Design review of the part built by this model. Coordinates are the model's own, in mm. Round coordinates to 2 decimals unless told otherwise and drop trailing zeros. Loops run counter-clockwise (first coordinate to the right, second up) from the corner with the lowest first, then second, coordinate; pieces in that order, holes last. Notation, with made-up numbers: (42.5, 6) - (66.5, 6) arc R15 cw to (66.5, 21) - close; hole circle Ø7 at (-0.75, -34.75). An arc over 180 degrees is marked (long way). Use one line per item in the form item = value. Start each with the question number.
(1) We need section B-B, the plane x = 52.5. Write out the cut boundary in (y, z), then the cut area to 3 significant figures.
(2) We need section D-D, the plane y = 1.5. Write out the cut boundary in (x, z).
(3) We need section A-A, the plane z = 45. Write out the cut boundary in (x, y), then the cut area to 3 significant figures.
(4) We need section C-C, the plane x = 0. Write out the cut boundary in (y, z).
(5) For pin 1 (5 mm diameter, centred on x = 52.5, z = 30.31, fed in from +Y); pin 2 (1.5 mm diameter, centred on x = -12.5, y = 2, fed in from -Z); pin 3 (1.5 mm diameter, centred on x = 37.5, y = 0.5, fed in from -Z), all flat-tipped, find the tip position at first contact; note any pin that passes through.
(6) Wall thickness on probe 1 along X at (y, z) = (1.75, -4); probe 2 along Z at (x, y) = (32, 2.35); probe 3 along Z at (x, y) = (-6, 2): over which ranges is each line inside the solid? List them lowest first. Write a range as [from, to].
from build123d import *

# Parameters (mm, degrees)
SKETCH1_R           = 3.05
SKETCH1_R_2         = 4
BOSS_EXTRUDE1_DEPTH = 3


with BuildPart() as part:
    # Sketch1 → Boss-Extrude1 (new body)
    with BuildSketch(Plane(origin=(0, 0, 0), x_dir=(1, 0, 0), z_dir=(0, 1, 0))):
        with BuildLine():
            Line((6.495190528, 64.371778265), (58.995190528, -26.560889132))
            ThreePointArc((58.995190528, -26.560889132), (58.995190528, -34.060889132), (52.5, -37.810889132))
            Line((52.5, -37.810889132), (-52.5, -37.810889132))
            ThreePointArc((-52.5, -37.810889132), (-58.995190528, -34.060889132), (-58.995190528, -26.560889132))
            Line((-58.995190528, -26.560889132), (-6.495190528, 64.371778265))
            ThreePointArc((-6.495190528, 64.371778265), (0, 68.121778265), (6.495190528, 64.371778265))
        make_face()
        with Locations((-52.5, -30.310889132)):
            Circle(SKETCH1_R, mode=Mode.SUBTRACT)
        with Locations((52.5, -30.310889132)):
            Circle(SKETCH1_R, mode=Mode.SUBTRACT)
        with Locations((0, 60.621778265)):
            Circle(SKETCH1_R, mode=Mode.SUBTRACT)
        with BuildLine():
            ThreePointArc((-52.5, -37.810889132), (-53.69003782, -37.715874614), (-54.849923408, -37.433238462))
            Line((-54.849923408, -37.433238462), (-3.133231211, -54.496465773))
            ThreePointArc((-3.133231211, -54.496465773), (0, -55), (3.133231211, -54.496465773))
            Line((3.133231211, -54.496465773), (54.849923408, -37.433238462))
            ThreePointArc((54.849923408, -37.433238462), (53.69003782, -37.715874614), (52.5, -37.810889132))
            Line((52.5, -37.810889132), (-52.5, -37.810889132))
        make_face()
        with Locations((0, -45)):
            Circle(SKETCH1_R_2, mode=Mode.SUBTRACT)
    extrude(amount=BOSS_EXTRUDE1_DEPTH)


solid = part.part
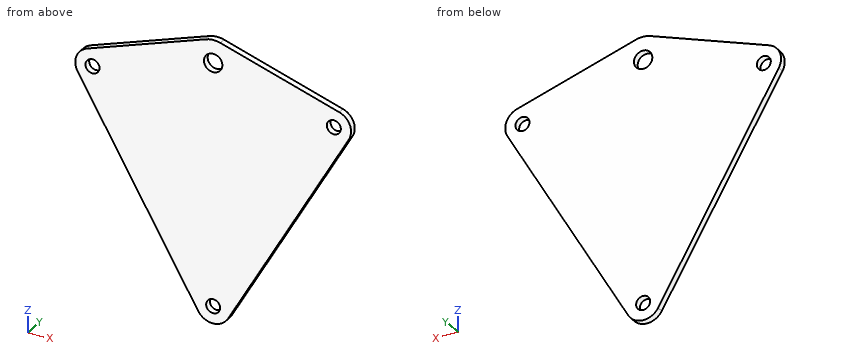
Data:
q1.outline = (0, 15.31) - (3, 15.31) - (3, 27.26) - (0, 27.26) - close; (0, 33.36) - (3, 33.36) - (3, 38.21) - (0, 38.21) - close
q1.area = 50.4 mm^2
q2.outline = (-59, 26.56) - (-6.5, -64.37) arc R7.5 ccw to (6.5, -64.37) - (59, 26.56) arc R7.5 ccw to (54.85, 37.43) - (3.13, 54.5) arc R10 ccw to (-3.13, 54.5) - (-54.85, 37.43) arc R7.5 ccw to start; hole circle Ø6.1 at (-52.5, 30.31); hole circle Ø8 at (0, 45); hole circle Ø6.1 at (0, -60.62); hole circle Ø6.1 at (52.5, 30.31)
q3.outline = (-31.92, 0) - (-4, 0) - (-4, 3) - (-31.92, 3) - close; (4, 0) - (31.92, 0) - (31.92, 3) - (4, 3) - close
q3.area = 167 mm^2
q4.outline = (0, -68.12) - (3, -68.12) - (3, -63.67) - (0, -63.67) - close; (0, -57.57) - (3, -57.57) - (3, 41) - (0, 41) - close; (0, 49) - (3, 49) - (3, 55) - (0, 55) - close
q5.pin_1 = through
q5.pin_2 = -55.27
q5.pin_3 = -11.97
q6.probe_1 = [-41.35, 41.35]
q6.probe_2 = [-20.2, 44.97]
q6.probe_3 = [-65.12, 53.55]
